Part model, mm, in its own coordinate system. Face numbers are marked on the shaded views. A direction names the side the tool comes from. Give positions to 0.01 mm unless a question says otherwise; leave off trailing zeros. Order: outer loops, then holes, each group sorted by start corner. A loop starts at its lowest first (then second) coordinate and runs counter-clockwise, first axis right, second up. Notation, with made-up numbers: M -5,1 L 33,1 A19 ccw 33,11 Z; hole C 1,-14.5 d3. An arc over 180 degrees is marked long. Answer as a JSON object with one key per item and string values.
from build123d import *

# Parameters (mm, degrees)
SCHIZZO1_R                   = 40
ESTRUSIONE_ESTRUSIONE1_DEPTH = 45
SCHIZZO2_W                   = 156
SCHIZZO2_H                   = 140
SCHIZZO2_R                   = 30
ESTRUSIONE_ESTRUSIONE2_DEPTH = 25
ESTRUSIONE_ESTRUSIONE4_DEPTH = 10
SCHIZZO6_W                   = 45
SCHIZZO6_H                   = 15
TAGLIO_ESTRUSIONE1_DEPTH     = 25


with BuildPart() as part:
    # Schizzo1 → Estrusione-Estrusione1 (new body)
    with BuildSketch(Plane(origin=(0, 0, 0), x_dir=(0, 0, -1), z_dir=(1, 0, 0))):
        with BuildLine():
            Line((-70, 0), (-70, 136.8))
            Line((-70, 136.8), (70, 136.8))
            Line((70, 136.8), (70, 0))
            ThreePointArc((70, 0), (0, -70), (-70, 0))
        make_face()
        with Locations(Location((0, 0, 0), (0, 0, 180))):
            Circle(SCHIZZO1_R, mode=Mode.SUBTRACT)
    extrude(amount=ESTRUSIONE_ESTRUSIONE1_DEPTH)

    # Schizzo2 → Estrusione-Estrusione2 (add)
    with BuildSketch(Plane(origin=(0, 136.8, 0), x_dir=(1, 0, 0), z_dir=(0, 1, 0))):
        with Locations((78, 0)):
            Rectangle(SCHIZZO2_W, SCHIZZO2_H)
        with Locations(Location((93.7, 0, 0), (0, 0, 270))):
            Circle(SCHIZZO2_R, mode=Mode.SUBTRACT)
    extrude(amount=ESTRUSIONE_ESTRUSIONE2_DEPTH)

    # Schizzo5 → Estrusione-Estrusione4 (add)
    with BuildSketch(Plane(origin=(0, 161.8, 0), x_dir=(1, 0, 0), z_dir=(0, 1, 0))):
        Polygon((156, 170), (156, 70), (0, 70), (0, -70), (-44, -70), (-44, 170), align=None)
    extrude(amount=-ESTRUSIONE_ESTRUSIONE4_DEPTH)

    # Schizzo6 → Taglio-Estrusione1 (cut)
    with BuildSketch(Plane(origin=(0, 161.8, 0), x_dir=(1, 0, 0), z_dir=(0, 1, 0))):
        with Locations((116.2, 0)):
            Rectangle(SCHIZZO6_W, SCHIZZO6_H)
    extrude(amount=-TAGLIO_ESTRUSIONE1_DEPTH, mode=Mode.SUBTRACT)


solid = part.part
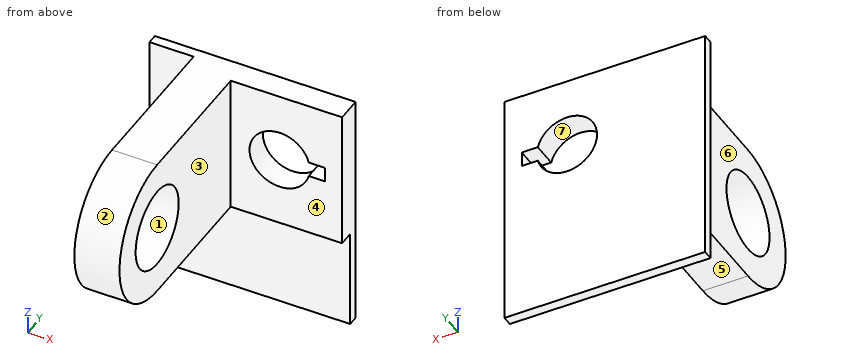
1. Cut at A-A on x = 93.7. Give the cut face in (y, z), plus the area to 3 significant figures.
Worked answers:
{"outline": "M 136.8,-70 L 151.8,-70 L 151.8,-170 L 161.8,-170 L 161.8,-30 L 136.8,-30 Z; M 136.8,30 L 161.8,30 L 161.8,70 L 136.8,70 Z", "area": "3,000 mm^2"}
2. Cut at C-C on x = 19. Give the cut face in (y, z).
Worked answers:
{"outline": "M 0,-70 L 151.8,-70 L 151.8,-170 L 161.8,-170 L 161.8,70 L 0,70 A70 ccw Z; hole C 0,0 d80"}
3. Probe line 1 along Z through (x, y) = (93.7, 148.75); line 2 along X through (y, z) = (155, 0); line 3 along Y through (x, z) = (-34, -123). List the from-to ranges inside material, lowest first.
Worked answers:
{"line 1": "z = -70 to -30, 30 to 70", "line 2": "x = -44 to 63.7, 138.7 to 156", "line 3": "y = 151.8 to 161.8"}
4. Two-plate mould, pull along Y, no slides. Class the marked faces 1, 2 and 3: +Y half, -Y half, draft (parallel to the pull), parting line (faces both ways), or undercut.
Worked answers:
{"face 1": "undercut", "face 2": "-Y half", "face 3": "draft"}
5. Cut at B-B on z = 0. Give the cut face in (x, y).
Worked answers:
{"outline": "M -44,151.8 L 0,151.8 L 0,40 L 45,40 L 45,136.8 L 63.7,136.8 L 63.7,161.8 L -44,161.8 Z; M 0,-70 L 45,-70 L 45,-40 L 0,-40 Z; M 138.7,136.8 L 156,136.8 L 156,161.8 L 138.7,161.8 Z"}
6. Pin check, flat tips, straight feed: P1, Ø1.5, axis at y = 5.5, z = -62.5, coming from the +X side; P2, Ø5, axis at y = -39.5, z = 26.5, coming from the -X side; P3, Ø1.5, axis at x = 20.5, z = 31, coming from the -Y side; P4, Ø8, axis at x = 131, y = 148.5, coming from the -Z side. Stop position of each tip, or through.
Worked answers:
{"P1": "stops at x = 45", "P2": "stops at x = 0", "P3": "stops at y = -63.13", "P4": "stops at z = -170"}
7. Which spindle directions (+Z, -Z, +X, -X, +Y, -Y) get a long thin tool onto all of the face, cutting with end or side? Do the marked faces 4, 5, 6 and 7. Say none if no direction does.
Worked answers:
{"face 4": "+Z, -Z, +X, -Y", "face 5": "-Z, +X, -X, -Y", "face 6": "+Z, -Z, -X, -Y", "face 7": "+Y, -Y"}
8. Cut at D-D on z = -56. Give the cut face in (x, y), plus the area to 3 significant figures.
Worked answers:
{"outline": "M -44,151.8 L 0,151.8 L 0,-42 L 45,-42 L 45,136.8 L 156,136.8 L 156,161.8 L -44,161.8 Z", "area": "12,400 mm^2"}
